from build123d import *

# Parameters (mm, degrees)
SKETCH2_R          = 6.5
CUT_EXTRUDE1_DEPTH = 0.75
SKETCH3_R          = 2.5
CUT_EXTRUDE2_DEPTH = 65.75
SKETCH5_R          = 3
CUT_EXTRUDE6_DEPTH = 19
CHAMFER1_SIZE      = 0.5
FILLET1_R          = 1


with BuildPart() as part:
    # Sketch1 → Revolve1 (revolve)
    with BuildSketch(Plane.XY, mode=Mode.PRIVATE) as revolve1_sk:
        with BuildLine():
            Line((0, 17), (0, 10.286668621))
            ThreePointArc((0, 10.286668621), (5.42509601, 7.238924157), (7.576230068, 1.4))
            Line((7.576230068, 1.4), (7.576230068, 0))
            Line((7.576230068, 0), (9.5, 0))
            Line((9.5, 0), (9.5, 13))
            Line((9.5, 13), (14.616013263, 13))
            Line((14.616013263, 13), (14.616013263, 15.037207554))
            ThreePointArc((14.616013263, 15.037207554), (14.160029693, 16.308432657), (13, 17))
            Line((13, 17), (0, 17))
        make_face()
    revolve(revolve1_sk.sketch.rotate(Axis((0, 0, 0), (0, 1, 0)), 90), axis=Axis((0, 0, 0), (0, 1, 0)))

    # Sketch2 → Cut-Extrude1 (cut)
    with BuildSketch(Plane(origin=(0, 17, 0), x_dir=(1, 0, 0), z_dir=(0, 1, 0))):
        with Locations(Location((0, 0, 0), (0, 0, 270))):
            Circle(SKETCH2_R)
    extrude(amount=-CUT_EXTRUDE1_DEPTH, mode=Mode.SUBTRACT)

    # Sketch3 → Cut-Extrude2 (cut)
    with BuildSketch(Plane(origin=(0, 16.25, 0), x_dir=(1, 0, 0), z_dir=(0, 1, 0))):
        with Locations(Location((0, 0, 0), (0, 0, 270))):
            Circle(SKETCH3_R)
    extrude(amount=-CUT_EXTRUDE2_DEPTH, mode=Mode.SUBTRACT)

    # Sketch5 → Cut-Extrude6 (cut)
    with BuildSketch(Plane(origin=(0, -8, 0), x_dir=(1, 0, 0), z_dir=(0, 1, 0))):
        with Locations(Location((0, 0, 0), (0, 0, 90))):
            Circle(SKETCH5_R)
    extrude(amount=CUT_EXTRUDE6_DEPTH, mode=Mode.SUBTRACT)

    # Chamfer1
    chamfer1_edges = [part.edges().sort_by_distance(p)[0] for p in [
        (0, 0, 9.5),
    ]]
    chamfer(chamfer1_edges, length=CHAMFER1_SIZE)

    # Fillet1
    # the kernel refuses this fillet: 1 mm, written as the material it adds along each edge
    with BuildSketch(Plane(origin=(0, 11, 0), x_dir=(0, 0, -1), z_dir=(1, 0, 0))) as fillet1_piece_1:
        with BuildLine():
            CenterArc((2, -0.866025404), FILLET1_R, 0, 60)
            Line((2.5, 0), (3, 0))
            Line((3, 0), (3, -0.866025404))
        make_face()
    revolve(axis=Axis((0, 11, 0), (0, 1, 0)))
    # the kernel refuses this fillet: 1 mm, written as the material it takes off along each edge
    with BuildSketch(Plane(origin=(0, 16.25, 0), x_dir=(0, 0, 1), z_dir=(-1, 0, 0))) as fillet1_2_piece_1:
        with BuildLine():
            CenterArc((2.5 + FILLET1_R, -FILLET1_R), FILLET1_R, 90, 90)
            Line((2.5 + FILLET1_R, 0), (2.5, 0))
            Line((2.5, 0), (2.5, -FILLET1_R))
        make_face()
    revolve(axis=Axis((0, 16.25, 0), (0, 1, 0)), mode=Mode.SUBTRACT)


solid = part.part
For this review, take the finished solid that the model builds, in its own axes (mm). A direction names the side the tool comes from. Round coordinates to 2 decimals unless told otherwise and drop trailing zeros. Use one line per item in the form item = value.
Item 1: Mouldability with a two-part tool opening along X and no side actions: class faces 1 (the cylindrical face through (7.396, 0.69, 1.642)), 2 (the flat face through (-3, 16.25, 3)), 3 (the flat face through (-6, 17, -3)), 4 (the cylindrical face through (14.27, 14.03, 3.17)) as +X half, -X half, draft (parallel to the pull), parting line (faces both ways), or undercut.
Answers:
face_1 = undercut
face_2 = undercut
face_3 = draft
face_4 = parting line
Item 2: Clearance check with flat-ended pins moving along their axes: P1, Ø1, axis at y = 10, z = 0, coming from the +X side; P2, Ø4, axis at x = -5, y = 3.5, coming from the -Z side; P3, Ø13.5, axis at x = 0, z = 0, coming from the -Y side. State where each tip first meets the part, or that it passes through.
Answers:
P1 = 9.5
P2 = -9.01
P3 = 5.17
Item 3: Tool access review of faces 5 (the flat face through (6, 0, -5)), 6 (the cylindrical face through (9.274, 6.838, 2.059)), 7 (the cylindrical face through (-3.955, 16.63, -5.158)): name each direction out of +Z, -Z, +X, -X, +Y, -Y from which nothing blocks a thin tool from reaching the whole face with its end or side.
Answers:
face_5 = +Z, -Z, +X, -X, -Y
face_6 = -Y
face_7 = +Y
Item 4: For line 1 (X direction, y = 13.9, z = 0); line 2 (X direction, y = 12.05, z = 0); line 3 (Y direction, x = 5.5, z = 10.5), list the stretches that pass through material, from the lowest coordinate up.
Answers:
line_1 = -14.62 to -2.5, 2.5 to 14.62
line_2 = -9.5 to -2.5, 2.5 to 9.5
line_3 = 13 to 17
